Geometry check sheet. Reference: the model listing, model coordinates, mm. Face numbers are marked on the shaded views. A direction names the side the tool comes from. Give positions to 0.01 mm unless a question says otherwise; leave off trailing zeros. Write each loop counter-clockwise with the first axis right and the second up, starting at its lowest first coordinate (ties: lowest second). Pieces come first, ordered by that corner, then holes. Notation, with made-up numbers: (78, 51.25) - (85, 51.25) arc R4 ccw to (85, 57.25) - close; hole circle Ø10 at (29.25, -30). An arc over 180 degrees is marked (long way). Use a Markdown table: item, result.
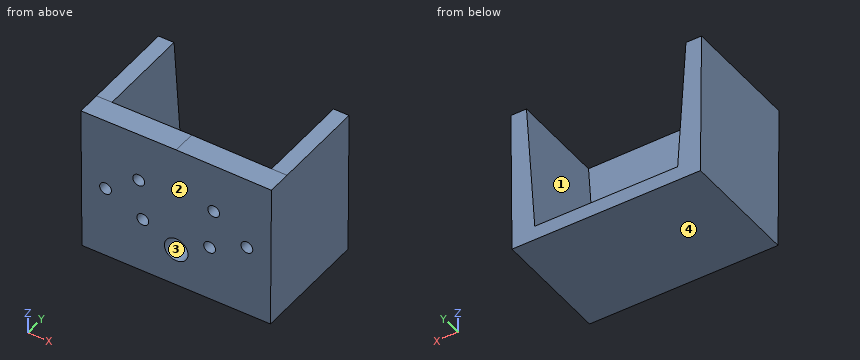
```python
from build123d import *
from build123d import SkipClean  # not in build123d's __all__

# Parameters (mm, degrees)
F1_DEPTH = 20
F3_DEPTH = 5
F4_D     = 2.5
F4_DEPTH = 5.001


with BuildPart() as f1:
    # F0 (on Front) → F1 (new body)
    with BuildSketch(Plane.XZ):
        Polygon((-19.9654586613, 0), (0, 0), (0, 3.0716089532), (-15.1386437938, 3.0716089532), (-16.8938487768, 30.7160895318), (-20.1848596334, 30.7160895318), align=None)
    extrude(amount=F1_DEPTH)

    # F2 (on face) → F3 (join)
    with BuildSketch(Plane.XZ.offset(20)):
        with BuildLine():
            Line((0, 30.8602673192), (-20.1848596334, 30.7160895318))
            Line((-20.1848596334, 30.7160895318), (-16.8938487768, 30.7160895318))
            Line((-16.8938487768, 30.7160895318), (-15.1386437938, 3.0716089532))
            Line((-15.1386437938, 3.0716089532), (0, 3.0716089532))
            Line((0, 3.0716089532), (0, 5.4992720857))
            ThreePointArc((0, 5.4992720857), (-2.5, 7.9992720857), (0, 10.4992720857))
            Line((0, 10.4992720857), (0, 30.8602673192))
        make_face()
        Polygon((-16.8938487768, 30.7160895318), (-20.1848596334, 30.7160895318), (-19.9654586613, 0), (0, 0), (0, 3.0716089532), (-15.1386437938, 3.0716089532), align=None)
    extrude(amount=F3_DEPTH)

    # F4 (through all, one way)
    with BuildSketch(Plane(origin=(0, -20, 0), x_dir=(1, 0, 0), z_dir=(0, 1, 0))):
        with Locations((-14.9744828703, -15.2839560666), (-7.0758488149, -11.7326774155), (-7.9496683148, -20.3487344883)):
            Circle(F4_D / 2)
    extrude(amount=-F4_DEPTH, mode=Mode.SUBTRACT)

    # F5: F1 across plane


with BuildPart() as f1_1:
    add(f1.part, clean=False)
    with SkipClean():  # cleaning this boolean's faces spoils the solid; the shape is the same uncleaned
        add(f1.part.mirror(Plane.YZ), clean=False)


solid = f1_1.part
```
1) Section check D-D on z = 10. Record the boundary of the cut face in (x, y), then the cut area to 3 significant figures.
Working result:
| item | result |
|---|---|
| outline | (-20.04, -25) - (-1.5, -25) - (-1.5, -20) - (-15.58, -20) - (-15.58, 0) - (-20.04, 0) - close; (1.5, -25) - (20.04, -25) - (20.04, 0) - (15.58, 0) - (15.58, -20) - (1.5, -20) - close |
| area | 364 mm² |
2) Depth check by flat-ended pin: P1, Ø5, axis at y = -9.5, z = 6, coming from the +X side; P2, Ø8.5, axis at x = -2, z = 17.5, coming from the +Y side; P3, Ø1, axis at x = -18, y = -15, coming from the +Z side; P4, Ø10, axis at x = -13.5, y = -6.5, coming from the -Z side. Enter the tip coordinate at first touch or a pass-through.
Working result:
| item | result |
|---|---|
| P1 | stops at x = 20.03 |
| P2 | stops at y = -20 |
| P3 | stops at z = 30.72 |
| P4 | stops at z = 0 |
3) Section check B-B on y = -22. Record the boundary of the cut face in (x, z).
Working result:
| item | result |
|---|---|
| outline | (-20.18, 30.72) - (-19.97, 0) - (19.97, 0) - (20.18, 30.72) - (0, 30.86) - close; hole circle Ø2.5 at (-14.97, 15.28); hole circle Ø2.5 at (-7.95, 20.35); hole circle Ø2.5 at (-7.08, 11.73); hole circle Ø5 at (0, 8); hole circle Ø2.5 at (7.08, 11.73); hole circle Ø2.5 at (7.95, 20.35); hole circle Ø2.5 at (14.97, 15.28) |
4) Set-up check for the marked faces 1 and 2: record each of +Z, -Z, +X, -X, +Y, -Y from which the full face is reachable in a straight line by a thin tool's end or side.
Working result:
| item | result |
|---|---|
| face 1 | +Z, +Y |
| face 2 | +Z, -Z, +X, -X, -Y |
5) Section check A-A on z = 21. Record the boundary of the cut face in (x, y), then the cut area to 3 significant figures.
Working result:
| item | result |
|---|---|
| outline | (-20.12, -25) - (-9.02, -25) - (-9.02, -20) - (-16.28, -20) - (-16.28, 0) - (-20.12, 0) - close; (-6.88, -25) - (6.88, -25) - (6.88, -20) - (-6.88, -20) - close; (9.02, -25) - (20.12, -25) - (20.12, 0) - (16.28, 0) - (16.28, -20) - (9.02, -20) - close |
| area | 333 mm² |
6) Section check C-C on x = 1.5. Record the boundary of the cut face in (y, z).
Working result:
| item | result |
|---|---|
| outline | (-25, 0) - (0, 0) - (0, 3.07) - (-20, 3.07) - (-20, 6) - (-25, 6) - close; (-25, 10) - (-20, 10) - (-20, 30.85) - (-25, 30.85) - close |
7) Mould release check, pull along X, two halves, no side actions. Record for the marked faces 3 and 4: pulls with the +X half, pulls with the -X half, needs draft (parallel to the pull), parting line crosses it, or undercut.
Working result:
| item | result |
|---|---|
| face 3 | undercut |
| face 4 | needs draft |
8) Material ranges on L1, parallel to X at y = -21.5, z = 11; L2, parallel to X at y = -22.75, z = 11.5; L3, parallel to Y at x = 3, z = 9.5, recorded low to high. Write a range as from..to.
Working result:
| item | result |
|---|---|
| L1 | x = -20.04..-8.09, -6.06..6.06, 8.09..20.04 |
| L2 | x = -20.05..-8.3, -5.85..5.85, 8.3..20.05 |
| L3 | y = -25..-20 |
